Work out the finished part from the listing and answer in its coordinate system (mm). A direction names the side the tool comes from. Give positions to 0.01 mm unless a question says otherwise; leave off trailing zeros. Order: outer loops, then holes, each group sorted by start corner. A loop starts at its lowest first (then second) coordinate and runs counter-clockwise, first axis right, second up. Notation, with made-up numbers: (29.25, -0.75) -> (53.25, -0.75) arc R21 cw to (53.25, 15.25) -> close; hole circle Ø2 at (42.5, 57). An arc over 180 degrees is marked (long way). Answer as CSV lines item,"result". Start each with the question number.
1. A cutting plane is placed at C-C (z = 5.65). Give the vertices of the cut face in (x, y), then the cut area to 3 significant figures.
2. For a pull along X with two mould halves and no side action, classify faces 3 (the cylindrical face through (-10.316, -7.91, 5.507)), 4 (the cylindrical face through (-11.5, 0.07, 5.51)), 5 (the flat face through (-2, 5, 0)) as released by +X, released by -X, zero draft, split by the parting line, or undercut.
3. A cutting plane is placed at A-A (x = 0). Give the vertices of the cut face in (y, z), then the cut area to 3 significant figures.
4. A cutting plane is placed at D-D (x = -10). Give the vertices of the cut face in (y, z).
5. For faces 1 (the flat face through (0, -6, 6)), 2 (the flat face through (6, -6, 5)), determine the directions among +Z, -Z, +X, -X, +Y, -Y from which every point of the face is accessible in a straight line to the end or side of a thin tool.
6. Find the intervals of material crossed by L1, parallel to Y at x = 0, z = 2; L2, parallel to Z at x = -7.25, y = 1.5; L3, parallel to Y at x = -10, z = 5.35, in increasing order.
7. Flat-ended cylindrical pins translate along their axes: pin 1 (3 mm diameter, centred on x = -6.5, z = 5, fed in from -Y); pin 2 (2 mm diameter, centred on y = 2.5, z = 2.5, fed in from -X); pin 3 (5 mm diameter, centred on x = 3.5, y = -10, fed in from -Z); pin 4 (2.5 mm diameter, centred on x = 10, y = 0, fed in from +Z). Find the tip coordinate at first contact, or state that the pin passes through.
8. A cutting plane is placed at B-B (y = 2). Give the vertices of the cut face in (x, z), then the cut area to 3 significant figures.
from build123d import *

# Parameters (mm, degrees)
SKETCH1_R           = 7
SKETCH1_R_2         = 5
BOSS_EXTRUDE1_DEPTH = 6
SKETCH2_R           = 13
SKETCH2_R_2         = 7
BOSS_EXTRUDE2_DEPTH = 1
SKETCH3_R           = 1.5
CUT_EXTRUDE1_DEPTH  = 1


with BuildPart() as part:
    # Sketch1 → Boss-Extrude1 (new body)
    with BuildSketch(Plane.XY):
        Circle(SKETCH1_R)
        Circle(SKETCH1_R_2, mode=Mode.SUBTRACT)
    extrude(amount=BOSS_EXTRUDE1_DEPTH)

    # Sketch2 → Boss-Extrude2 (add)
    with BuildSketch(Plane.XY.offset(6)):
        Circle(SKETCH2_R)
        Circle(SKETCH2_R_2, mode=Mode.SUBTRACT)
    extrude(amount=-BOSS_EXTRUDE2_DEPTH)

    # Sketch3 → Cut-Extrude1 (cut)
    with BuildSketch(Plane.XY.offset(6)):
        with Locations((-10, 0)):
            Circle(SKETCH3_R)
        with Locations((10, 0)):
            Circle(SKETCH3_R)
    extrude(amount=-CUT_EXTRUDE1_DEPTH, mode=Mode.SUBTRACT)


solid = part.part
Answer sheet:
1,outline,"circle Ø26 at (0, 0); hole circle Ø3 at (-10, 0); hole circle Ø10 at (0, 0); hole circle Ø3 at (10, 0)"
1,area,"438 mm^2"
2,face 3,"split by the parting line"
2,face 4,"undercut"
2,face 5,"zero draft"
3,outline,"(-13, 5) -> (-7, 5) -> (-7, 0) -> (-5, 0) -> (-5, 6) -> (-13, 6) -> close; (5, 0) -> (7, 0) -> (7, 5) -> (13, 5) -> (13, 6) -> (5, 6) -> close"
3,area,"36.0 mm^2"
4,outline,"(-8.31, 5) -> (-1.5, 5) -> (-1.5, 6) -> (-8.31, 6) -> close; (1.5, 5) -> (8.31, 5) -> (8.31, 6) -> (1.5, 6) -> close"
5,face 1,"+Z, +X, -X, +Y, -Y"
5,face 2,"-Z"
6,L1,"y = -7 to -5, 5 to 7"
6,L2,"z = 5 to 6"
6,L3,"y = -8.31 to -1.5, 1.5 to 8.31"
7,pin 1,"stops at y = -12"
7,pin 2,"stops at x = -6.84"
7,pin 3,"stops at z = 5"
7,pin 4,"passes through"
8,outline,"(-12.85, 5) -> (-6.71, 5) -> (-6.71, 0) -> (-4.58, 0) -> (-4.58, 6) -> (-12.85, 6) -> close; (4.58, 0) -> (6.71, 0) -> (6.71, 5) -> (12.85, 5) -> (12.85, 6) -> (4.58, 6) -> close"
8,area,"37.8 mm^2"
